Here's the drawing with two shaded views (mm, measured from the low corner). I have some questions. A direction names the side the tool comes from. Coordinates: 2 decimals unless noted, no trailing zeros. Order: outer loops, then holes, each group sorted by start corner. A loop starts at its lowest first (then second) coordinate and runs counter-clockwise, first axis right, second up. Notation, with made-up numbers: (0.5, -16.75) -> (57.5, -16.75) arc R28 cw to (57.5, 15.25) -> close; hole circle Ø4 at (33.5, 64). An arc over 180 degrees is marked (long way). One line per item, written item: value. Start each with the question number.
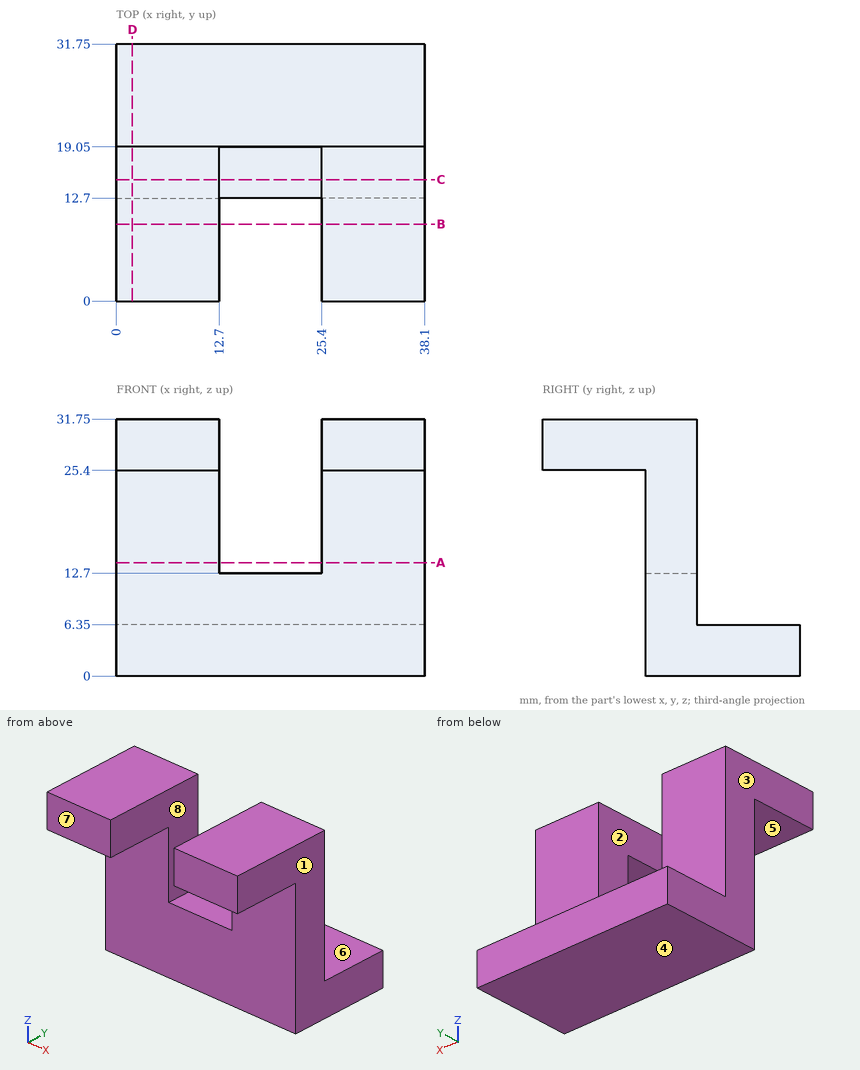
Q1. If we mould it in two halves opening along X, with no side actions, what happens to the marked faces 1, 2, 3 and 4? For each: +X half, -X half, draft (parallel to the pull), parting line (faces both ways), or undercut.
Q2. For the marked faces 5, 6, 7 and 8, which set-ups out of +Z, -Z, +X, -X, +Y, -Y let a thin tool reach every point of the face, with its end or its side?
Q3. Imagine slicing it at B-B (y = 9.5). Write out the boundary of the cut face in (x, z), plus the area to 3 significant figures.
Q4. Imagine slicing it at A-A (z = 14). Write out the boundary of the cut face in (x, y), plus the area to 3 significant figures.
Q5. Imagine slicing it at D-D (x = 2). Write out the boundary of the cut face in (y, z).
Q6. I need wall thicknesses on line 1 (Z direction, x = 37, y = 28.5); line 2 (Y direction, x = 23, z = 11); line 3 (Z direction, x = 8.5, y = 7). Which ranges of each line are inside material? Lowest first, please.
Q7. Imagine slicing it at C-C (y = 15). Write out the boundary of the cut face in (x, z), plus the area to 3 significant figures.
Q8. For P1, Ø2, axis at x = 16, y = 24, coming from the +Z side; P2, Ø12.5, axis at x = 26, z = 25.5, coming from the +Y side; P3, Ø3, axis at x = 11, z = 13, coming from the -Y side, each with a flat end and sliding along its axis, tell me the tip position at first contact or that it passes through.
Completed:
1. face 1: +X half
1. face 2: undercut
1. face 3: -X half
1. face 4: draft
2. face 5: -Z, +X, -X, -Y
2. face 6: +Z, +X, -X, +Y
2. face 7: +Z, -Z, +X, -X, -Y
2. face 8: +Z, +Y, -Y
3. outline: (0, 25.4) -> (12.7, 25.4) -> (12.7, 31.75) -> (0, 31.75) -> close; (25.4, 25.4) -> (38.1, 25.4) -> (38.1, 31.75) -> (25.4, 31.75) -> close
3. area: 161 mm2
4. outline: (0, 12.7) -> (12.7, 12.7) -> (12.7, 19.05) -> (0, 19.05) -> close; (25.4, 12.7) -> (38.1, 12.7) -> (38.1, 19.05) -> (25.4, 19.05) -> close
4. area: 161 mm2
5. outline: (0, 25.4) -> (12.7, 25.4) -> (12.7, 0) -> (31.75, 0) -> (31.75, 6.35) -> (19.05, 6.35) -> (19.05, 31.75) -> (0, 31.75) -> close
6. line 1: z = 0 to 6.35
6. line 2: y = 12.7 to 19.05
6. line 3: z = 25.4 to 31.75
7. outline: (0, 0) -> (38.1, 0) -> (38.1, 31.75) -> (25.4, 31.75) -> (25.4, 12.7) -> (12.7, 12.7) -> (12.7, 31.75) -> (0, 31.75) -> close
7. area: 968 mm2
8. P1: stops at z = 6.35
8. P2: stops at y = 19.05
8. P3: stops at y = 12.7
